Here's how the part is built. I have some questions about the finished solid (model axes, mm). Round coordinates to 2 decimals unless told otherwise and drop trailing zeros. Write each loop counter-clockwise with the first axis right and the second up, starting at its lowest first coordinate (ties: lowest second). Pieces come first, ordered by that corner, then holes. Notation, with made-up numbers: M 56.25,33.25 L 70.25,33.25 A27 cw 70.25,70.25 Z; hole C 38,77.5 d11. An arc over 180 degrees is marked long. Use one line per item in the form item = value. Start each with the question number.
Q1. I need wall thicknesses on line 1 along X through (y, z) = (0.8, 0); line 2 along Z through (x, y) = (12, 0.9); line 3 along X through (y, z) = (0.45, -0.5). Which ranges of each line are inside material? Lowest first, please. Write a range as from..to.
Q2. I want a section at D-D on z = -2.55. List the corners of the cut face in (x, y) for me, and give its area (3 significant figures).
Q3. I want a section at A-A on z = 0. List the corners of the cut face in (x, y) for me.
Q4. We'd pull the mould along X, two halves only. Please class faces 1 (the face through (0, 1, 3)), 2 (the face through (10.5, 1.01, -0.07)), 3 (the face through (15, 1, 0)), 4 (the face through (-13.5, 1.01, -0.07)): +X half, -X half, draft (parallel to the pull), parting line (faces both ways), or undercut.
Q5. I want a section at B-B on y = 1.2. List the corners of the cut face in (x, z) for me.
Q6. I want a section at C-C on z = 2.35. List the corners of the cut face in (x, y) for me, and give its area (3 significant figures).
Autodesk Inventor part; units mm, degrees
ref_plane "YZ Plane" through (0, 0, 0) normal (1, 0, 0) x (0, 1, 0)
ref_plane "XZ Plane" through (0, 0, 0) normal (0, 1, 0) x (-1, 0, 0)
ref_plane "XY Plane" through (0, 0, 0) normal (0, 0, 1) x (1, 0, 0)
sketch "Sketch1" plane through (0, 0, 0) normal (0, 1, 0) x (-1, 0, 0)
  line L0 (-12, -3) -> (12, -3)
  line L1 (12, -3) -> (12, 3)
  line L2 (12, 3) -> (-12, 3)
  line L3 (-12, 3) -> (-12, -3)
  line L4 (-12, -3) -> (12, 3) construction
  line L5 (12, -3) -> (-12, 3) construction
  circle A0 centre (12, 0) radius 3
  circle A1 centre (-12, 0) radius 3
  point P0 (0, 0)
  dimension "d0" = 24
  dimension "d1" = 6
  dimension "d2" = 6
  dimension "d3" = 6
extrude "Extrusion1" add sketch "Sketch1" along normal blind 2
sketch "Sketch2" plane through (0, 2, 0) normal (0, 1, 0) x (1, 0, 0)
  arc A0 (12, -3) -> (12, 3) centre (12, 0) ccw
  arc A1 (-12, 3) -> (-12, -3) centre (-12, 0) ccw
  circle A2 centre (-12, 0) radius 1
  circle A3 centre (12, 0) radius 1.5
  circle A4 centre (-12, 0) radius 1.5
  point P0 (0, 0)
  dimension "d6" = 2
  dimension "d7" = 3
  dimension "d8" = 3
extrude "Extrusion2" cut sketch "Sketch2" against normal blind 2 contours A2 | A3 | A4
properties part number "tahlo5"
Reported:
q1.line_1 = -15..-13.5, -10.5..10.5, 13.5..15
q1.line_2 = -3..-1.5, 1.5..3
q1.line_3 = -14.96..-13.41, -10.59..10.59, 13.41..14.96
q2.outline = M -13.58,0 L 13.58,0 L 13.58,2 L -13.58,2 Z
q2.area = 54.3 mm^2
q3.outline = M -15,0 L -13.5,0 L -13.5,2 L -15,2 Z; M -10.5,0 L 10.5,0 L 10.5,2 L -10.5,2 Z; M 13.5,0 L 15,0 L 15,2 L 13.5,2 Z
q4.face_1 = draft
q4.face_2 = undercut
q4.face_3 = +X half
q4.face_4 = undercut
q5.outline = M -12,-3 L 12,-3 A3 ccw 12,3 L -12,3 A3 ccw Z; hole C -12,0 d3; hole C 12,0 d3
q6.outline = M -13.86,0 L 13.86,0 L 13.86,2 L -13.86,2 Z
q6.area = 55.5 mm^2
